Work out the finished part from the listing and answer in its coordinate system (mm). A direction names the side the tool comes from. Round coordinates to 2 decimals unless told otherwise and drop trailing zeros. Loops run counter-clockwise (first coordinate to the right, second up) from the corner with the lowest first, then second, coordinate; pieces in that order, holes last.
```python
from build123d import *

# Parameters (mm, degrees)
EXTRUDE6_DEPTH               = 32
EXTRUDE13_DEPTH              = 22
SKETCH12_R                   = 6
EXTRUDE14_DEPTH              = 22
F_6_0_6_DIAMETER_HOLE1_D     = 6
F_6_0_6_DIAMETER_HOLE1_DEPTH = 16
F_6_0_6_DIAMETER_HOLE1_TIP   = 1.802581857


# Read off the part's stored shape, not the designer's step: CBORE for M6 Hex Head Bolt1
with BuildPart() as part:
    # Sketch8 → Extrude6 (new body)
    with BuildSketch(Plane.XY):
        Polygon((-78.603037361, 32.929005068), (-54.603037361, 32.929005068), (-54.603037361, 23.929005068), (-38.603037361, 23.929005068), (-38.603037361, 32.929005068), (-14.603037361, 32.929005068), (-14.603037361, 68.929005068), (-78.603037361, 68.929005068), align=None)
    extrude(amount=-EXTRUDE6_DEPTH)

    # Sketch9 → Extrude13 (cut)
    with BuildSketch(Plane.XY):
        with BuildLine():
            Line((-73.272586686, 44.123559999), (-59.381205522, 62.558045439))
            ThreePointArc((-59.381205522, 62.558045439), (-53.742202371, 67.247954854), (-46.603037361, 68.929005068))
            Line((-46.603037361, 68.929005068), (-78.603037361, 68.929005068))
            Line((-78.603037361, 68.929005068), (-78.603037361, 42.929005068))
            Line((-78.603037361, 42.929005068), (-75.668493217, 42.929005068))
            ThreePointArc((-75.668493217, 42.929005068), (-74.329899777, 43.244201983), (-73.272586686, 44.123559999))
        make_face()
        with BuildLine():
            Line((-14.603037361, 68.929005068), (-46.603037361, 68.929005068))
            ThreePointArc((-46.603037361, 68.929005068), (-39.463872351, 67.247954854), (-33.8248692, 62.558045439))
            Line((-33.8248692, 62.558045439), (-19.933488035, 44.123559999))
            ThreePointArc((-19.933488035, 44.123559999), (-18.876174944, 43.244201983), (-17.537581505, 42.929005068))
            Line((-17.537581505, 42.929005068), (-14.603037361, 42.929005068))
            Line((-14.603037361, 42.929005068), (-14.603037361, 68.929005068))
        make_face()
    extrude(amount=-EXTRUDE13_DEPTH, mode=Mode.SUBTRACT)

    # Sketch12 → Extrude14 (cut)
    with BuildSketch(Plane.XY):
        with Locations((-46.603037361, 52.929005068)):
            Circle(SKETCH12_R)
    extrude(amount=-EXTRUDE14_DEPTH, mode=Mode.SUBTRACT)

    # Ø6.0 (6) Diameter Hole1
    with Locations(Plane(origin=(-46.603037361, 23.929005068, -8), x_dir=(0, 0, -1), z_dir=(0, -1, 0))):
        with Locations((0, 0), (16, 0)):
            Hole(F_6_0_6_DIAMETER_HOLE1_D / 2, depth=F_6_0_6_DIAMETER_HOLE1_DEPTH)
            with Locations((0, 0, -(F_6_0_6_DIAMETER_HOLE1_DEPTH + F_6_0_6_DIAMETER_HOLE1_TIP / 2))):  # 118° drill point
                Cone(0, F_6_0_6_DIAMETER_HOLE1_D / 2, F_6_0_6_DIAMETER_HOLE1_TIP, mode=Mode.SUBTRACT)

    # CBORE for M6 Hex Head Bolt1 outline → CBORE for M6 Hex Head Bolt1 (revolve, cut)
    with BuildSketch(Plane(origin=(-49.700366285, 3.088627955, -12.000023726), x_dir=(0.9980745763174489, -0.06202531828813871, 0), z_dir=(0, 0, 1))):
        Polygon((0, 54.947204966), (3.3, 54.947204966), (3.3, 61.556526083), (7.275, 61.556526083), (7.275, 65.936761667), (0, 65.936761667), align=None)
    revolve(axis=Axis((-49.700366285, 3.088627955, -12.000023726), (0.062025318288138724, 0.9980745763174491, 0)), mode=Mode.SUBTRACT)


solid = part.part
```
1. Find section A-A (z = -28.5). Write down the section's boundary in (x, y).
Answer key:
outline: (-78.6, 32.93) - (-54.6, 32.93) - (-54.6, 23.93) - (-38.6, 23.93) - (-38.6, 32.93) - (-14.6, 32.93) - (-14.6, 68.93) - (-78.6, 68.93) - close
2. Find section C-C (y = 36.5). Write down the section's boundary in (x, z), then the cut area to 3 significant figures.
Answer key:
outline: (-78.6, -32) - (-14.6, -32) - (-14.6, 0) - (-78.6, 0) - close; hole circle Ø6 at (-46.6, -24); hole circle Ø6 at (-46.6, -8)
area: 1,990 mm2
3. Determine the mould class of faces 4 (the face through (-47.1, 46.7, 0)), 5 (the face through (-77, 42.929, -11)), 6 (the face through (-46.92, 41.42, -23.59)) for opening direction Z: +Z half, -Z half, draft (parallel to the pull), parting line (faces both ways), or undercut.
Answer key:
face 4: +Z half
face 5: draft
face 6: undercut
4. Find section D-D (y = 48.5). Write down the section's boundary in (x, z).
Answer key:
outline: (-78.6, -32) - (-14.6, -32) - (-14.6, -22) - (-23.23, -22) - (-23.23, 0) - (-42.56, 0) - (-42.56, -22) - (-50.65, -22) - (-50.65, 0) - (-69.97, 0) - (-69.97, -22) - (-78.6, -22) - close
5. Find section B-B (x = -24). Write down the section's boundary in (y, z).
Answer key:
outline: (32.93, -32) - (68.93, -32) - (68.93, -22) - (49.52, -22) - (49.52, 0) - (32.93, 0) - close
6. Which of the six approach directions +Z, -Z, +X, -X, +Y, -Y give full straight-line access (tool end or side, diameter ignored) to faces 1 (the face through (-49.53, 32.04, -8.65)), 2 (the face through (-27, 53.5, -10.8)), 3 (the face through (-27, 32.929, -16))?
Answer key:
face 1: -Y
face 2: +Z, +X, +Y
face 3: +Z, -Z, +X, -Y
7. Consider probe 1 along X at (y, z) = (28.5, -8); probe 2 along Z at (x, y) = (-47, 35.5); probe 3 along X at (y, z) = (29.5, -19). Determine where each line is inside the solid, lowest interval first.
Answer key:
probe 1: x = -54.6 to -49.6, -43.6 to -38.6
probe 2: z = -32 to -26.97, -21.03 to -10.97, -5.03 to 0
probe 3: x = -54.6 to -38.6
8. Given pin 1 (2.5 mm diameter, centred on x = -16, z = -15.5, fed in from +Y); pin 2 (4 mm diameter, centred on y = 30.5, z = -3.5, fed in from +X); pin 3 (1.5 mm diameter, centred on x = -65, z = -23, fed in from -Y), each flat-ended and moving along its own axis, determine where each tip first touches the part or whether it passes through.
Answer key:
pin 1: stops at y = 42.93
pin 2: stops at x = -38.6
pin 3: stops at y = 32.93
